Here's the drawing with two shaded views (mm, measured from the low corner). I have some questions. A direction names the side the tool comes from. Give positions to 0.01 mm unless a question says otherwise; leave off trailing zeros. Write each loop counter-clockwise with the first axis right and the second up, starting at its lowest first coordinate (ties: lowest second). Pieces come first, ordered by that corner, then holes. Notation, with made-up numbers: (26, -14.75) - (37, -14.75) arc R12 cw to (37, -5.75) - close; hole circle Ø9 at (79, 40.25). An arc over 180 degrees is marked (long way). Write item = value, one per line.
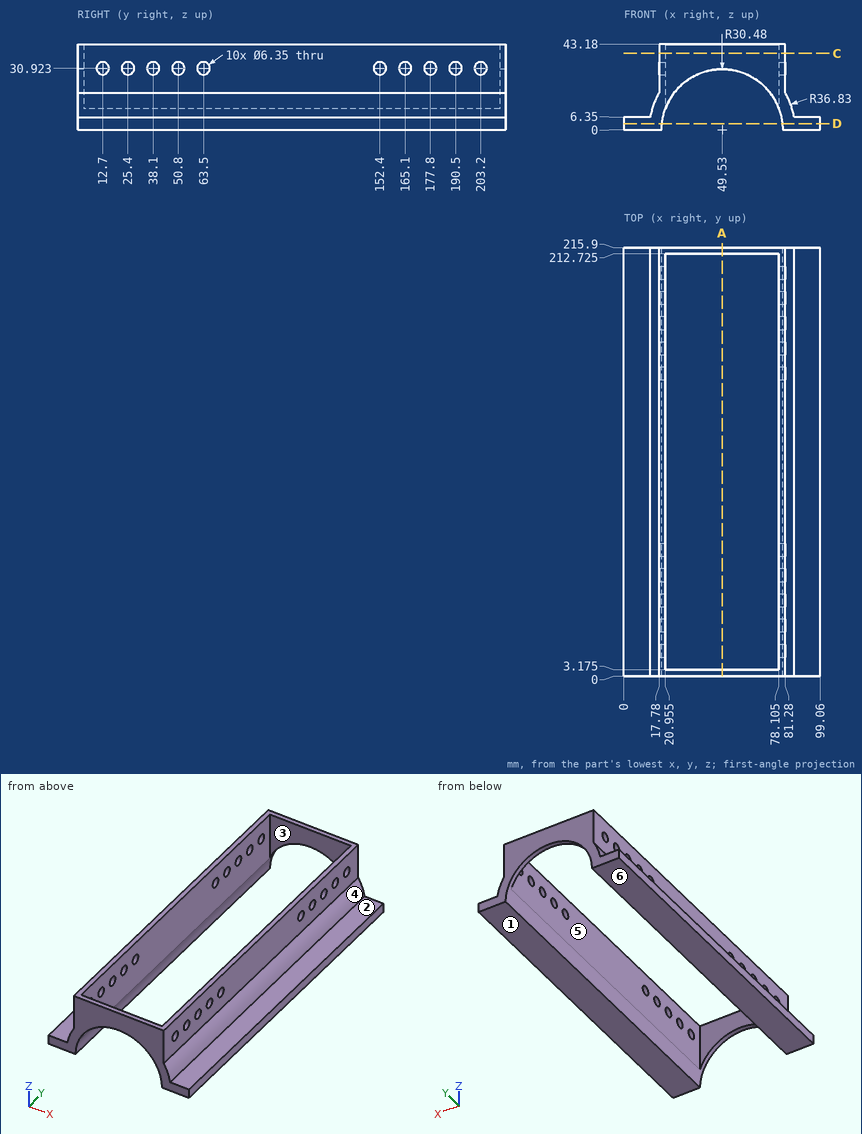
1. If we section it at D-D, the plane z = 3: Please give me the cut outline in (x, y), and give its area (3 significant figures).
Filled sheet:
outline = (0, 0) - (19.2, 0) - (19.2, 215.9) - (0, 215.9) - close; (79.86, 0) - (99.06, 0) - (99.06, 215.9) - (79.86, 215.9) - close
area = 8,290 mm2
2. If we section it at A-A, the plane x = 49.53: Please give me the cut outline in (y, z) (1 decimal).
Filled sheet:
outline = (0, 30.5) - (3.2, 30.5) - (3.2, 43.2) - (0, 43.2) - close; (212.7, 30.5) - (215.9, 30.5) - (215.9, 43.2) - (212.7, 43.2) - close
3. Thinking about a two-plate mould opening in X: for the marked faces 4, 5 and 6, which applies, pulls with the +X half, pulls with the -X half, needs draft (parallel to the pull), parting line crosses it, or undercut?
Filled sheet:
face_4 = pulls with the +X half
face_5 = undercut
face_6 = needs draft
4. Which directions (+Z, -Z, +X, -X, +Y, -Y) give clear straight access to the entire face, cutting with the end or side of a thin tool? Please do the marked faces 1, 2 and 3.
Filled sheet:
face_1 = -Z, +X, -X, +Y, -Y
face_2 = +Z, +X, +Y, -Y
face_3 = +Z, -Z
5. If we section it at C-C, the plane z = 38.5: Please give me the cut outline in (x, y) (1 decimal).
Filled sheet:
outline = (17.8, 0) - (81.3, 0) - (81.3, 215.9) - (17.8, 215.9) - close; hole (21, 3.2) - (78.1, 3.2) - (78.1, 212.7) - (21, 212.7) - close
6. For pin 1 (12.5 mm diameter, centred on y = 125.5, z = 26, fed in from -X); pin 2 (4 mm diameter, centred on y = 203.2, z = 30.92, fed in from +X); pin 3 (4 mm diameter, centred on x = 5, y = 103, fed in from +Z); pin 4 (10 mm diameter, centred on y = 50.8, z = 30.92, fed in from +X), each with a flat end and sliding along its axis, tell me the tip position at first contact or that it passes through.
Filled sheet:
pin_1 = 17.78
pin_2 = through
pin_3 = 6.35
pin_4 = 81.28
7. I need wall thicknesses on line 1 (Z direction, x = 18.95, y = 152.4); line 2 (Y direction, x = 37, z = 39) (1 decimal); line 3 (X direction, y = 43, z = 34.5) (1 decimal). Which ranges of each line are inside material? Lowest first, please.
Filled sheet:
line_1 = 0 to 27.75, 34.1 to 43.18
line_2 = 0 to 3.2, 212.7 to 215.9
line_3 = 17.8 to 21, 78.1 to 81.3
